from build123d import *

# Parameters (mm, degrees)
F1_DEPTH  = 8.89
F3_DEPTH  = 2.54
F5_DEPTH  = 2.54
F6_W      = 4.75
F6_H      = 6.159577
F8_W      = 4.75
F8_H      = 6.147177
F7_W      = 4.75
F7_H      = 6.147177
F9_W      = 4.75
F9_H      = 6.147177
F10_DEPTH = 6
F11_R     = 1.5
F12_R     = 1.5
F13_R     = 1.5
F14_R     = 1.5
F15_DEPTH = 6
F16_R     = 0.5
F17_DEPTH = 3.5


with BuildPart() as f1:
    # F0 (on Right) → F1 (new body, symmetric)
    with BuildSketch(Plane.YZ):
        Polygon((10.382133, 24.079738), (1.882133, 24.079738), (1, 19.076915), (0, 19.076915), (0, 12.679738), (-8.5, 12.679738), (-9.382133, 7.676915), (-10.382133, 7.676915), (-10.382133, 1.279738), (-18.882133, 1.279738), (-19.764265, -3.723085), (-20.764265, -3.723085), (-20.764265, -10.120262), (-29.264265, -10.120262), (-30.146398, -15.123085), (-31.146398, -15.123085), (-31.146398, -23.920262), (11.753602, -23.920262), (11.753602, 14.92088), align=None)
    extrude(amount=F1_DEPTH, both=True)

    # F2 (on face) → F3 (cut)
    with BuildSketch(Plane(origin=(-8.89, 0, 0), x_dir=(0, -1, 0), z_dir=(-1, 0, 0))):
        Polygon((-11.753602, -23.920262), (0, -23.920262), (0, 12.679738), (0, 19.076915), (-1, 19.076915), (-1.882133, 24.079738), (-10.382133, 24.079738), (-11.753602, 14.92088), align=None)
        Polygon((20.764265, -23.920262), (20.764265, -10.120262), (20.764265, -3.723085), (19.764265, -3.723085), (18.882133, 1.279738), (10.382133, 1.279738), (10.382133, -23.920262), align=None)
    extrude(amount=-F3_DEPTH, mode=Mode.SUBTRACT)

    # F4 (on face) → F5 (cut)
    with BuildSketch(Plane.YZ.offset(8.89)):
        Polygon((-20.764265, -23.920262), (-20.764265, -10.120262), (-29.264265, -10.120262), (-30.146398, -15.123085), (-31.146398, -15.123085), (-31.146398, -23.920262), align=None)
        Polygon((-10.382133, 1.279738), (-10.382133, -23.920262), (0, -23.920262), (0, 12.679738), (-8.5, 12.679738), (-9.382133, 7.676915), (-10.382133, 7.676915), align=None)
    extrude(amount=-F5_DEPTH, mode=Mode.SUBTRACT)

    # F6 (on face) + F8 (on face) + F7 (on face) + F9 (on face) → F10 (cut)
    with BuildSketch(Plane.XZ.offset(31.146398)):
        with Locations((-6.265, -18.452873)):
            Rectangle(F6_W, F6_H)
        with Locations((-1.265, -18.452873)):
            Rectangle(F6_W, F6_H)
        with Locations((3.735, -18.452873)):
            Rectangle(F6_W, F6_H)
    with BuildSketch(Plane.XZ.offset(10.382133)):
        Polygon((-8.64, 7.426915), (-8.64, 1.279738), (-6.35, 1.279738), (-3.89, 1.279738), (-3.89, 7.426915), align=None)
        with Locations((-1.265, 4.353326)):
            Rectangle(F8_W, F8_H)
        with Locations((3.735, 4.353326)):
            Rectangle(F8_W, F8_H)
    with BuildSketch(Plane.XZ.offset(20.764265)):
        with Locations((-3.725, -7.046673)):
            Rectangle(F7_W, F7_H)
        with Locations((1.275, -7.046673)):
            Rectangle(F7_W, F7_H)
        Polygon((3.9, -3.973085), (3.9, -10.120262), (6.35, -10.120262), (8.65, -10.120262), (8.65, -3.973085), align=None)
    with BuildSketch(Plane.XZ):
        with Locations((-3.725, 15.753327)):
            Rectangle(F9_W, F9_H)
        with Locations((1.275, 15.753327)):
            Rectangle(F9_W, F9_H)
        Polygon((3.9, 18.826915), (3.9, 12.679738), (6.35, 12.679738), (8.65, 12.679738), (8.65, 18.826915), align=None)
    extrude(amount=-F10_DEPTH, mode=Mode.SUBTRACT)

    # F11 (on face) + F12 (on face) + F13 (on face) + F14 (on face) → F15 (cut)
    with BuildSketch(Plane.XY.offset(-10.120262)):
        with Locations((-6.265, -27.264265)):
            Circle(F11_R)
        with Locations((-1.265, -27.264265)):
            Circle(F11_R)
        with Locations((3.735, -27.264265)):
            Circle(F11_R)
    with BuildSketch(Plane.XY.offset(1.279738)):
        with Locations((-3.725, -16.882133)):
            Circle(F12_R)
        with Locations((1.275, -16.882133)):
            Circle(F12_R)
        with Locations((6.275, -16.882133)):
            Circle(F12_R)
    with BuildSketch(Plane.XY.offset(12.679738)):
        with Locations((-6.265, -6.5)):
            Circle(F13_R)
        with Locations((-1.265, -6.5)):
            Circle(F13_R)
        with Locations((3.735, -6.5)):
            Circle(F13_R)
    with BuildSketch(Plane.XY.offset(24.079738)):
        with Locations((-3.725, 3.882133)):
            Circle(F14_R)
        with Locations((1.275, 3.882133)):
            Circle(F14_R)
        with Locations((6.275, 3.882133)):
            Circle(F14_R)
    extrude(amount=-F15_DEPTH, mode=Mode.SUBTRACT)

    # F16 (on face) → F17 (join)
    with BuildSketch(Plane(origin=(0, 0, -23.920262), x_dir=(1, 0, 0), z_dir=(0, 0, -1))):
        with Locations((3.81, 26.496398)):
            Circle(F16_R)
        with Locations((-1.27, 26.496398)):
            Circle(F16_R)
        with Locations((-6.35, 26.496398)):
            Circle(F16_R)
        with Locations((6.35, 11.256398)):
            Circle(F16_R)
        with Locations((1.27, 11.256398)):
            Circle(F16_R)
        with Locations((-3.81, 11.256398)):
            Circle(F16_R)
        with Locations((-6.35, 1.096398)):
            Circle(F16_R)
        with Locations((-1.27, 1.096398)):
            Circle(F16_R)
        with Locations((3.81, 1.096398)):
            Circle(F16_R)
        with Locations((6.35, -9.063602)):
            Circle(F16_R)
        with Locations((1.27, -9.063602)):
            Circle(F16_R)
        with Locations((-3.81, -9.063602)):
            Circle(F16_R)
    extrude(amount=F17_DEPTH)


solid = f1.part
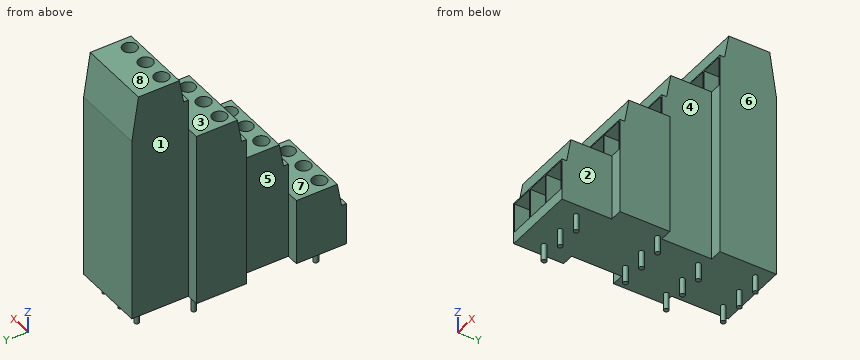
Check sheet for the modelled part. Datum: model origin and axes. Units: mm. Face numbers are marked on the shaded views. A direction names the side the tool comes from. Round coordinates to 2 decimals unless told otherwise and drop trailing zeros. Loops run counter-clockwise (first coordinate to the right, second up) from the corner with the lowest first, then second, coordinate; pieces in that order, holes last. Notation, with made-up numbers: (76, -29) - (82, -29) arc R24 ccw to (82, 3) - close; hole circle Ø5 at (70.25, 7). An arc over 180 degrees is marked (long way). Answer as CSV lines item,"result". Start each with the question number.
Item 1: Section check C-C (z = -20.5). Record the boundary of the cut face in (x, y), and give its area (3 significant figures).
Item 2: Set-up check for the marked faces 1, 2, 3, 4 and 5: record each of +Z, -Z, +X, -X, +Y, -Y from which the full face is reachable in a straight line by a thin tool's end or side.
Item 3: Scan lines: line 1 (X direction, y = -27, z = -16); line 2 (X direction, y = 4.5, z = 16.5); line 3 (Z direction, x = 5.5, y = 2). Record each from-to range of solid material in increasing order. Write a range as [from, to].
Item 4: Section check D-D (z = 6.5). Record the boundary of the cut face in (x, y), and give its area (3 significant figures).
Item 5: Section check A-A (y = -6.5). Record the boundary of the cut face in (x, z) (3 decimals), and give its area (3 significant figures).
Item 6: Depth check by flat-ended pin: P1, Ø1.8, axis at x = -6.26, y = -27.26, coming from the +Z side; P2, Ø4, axis at x = 2.5, y = -29.5, coming from the +Z side; P3, Ø0.5, axis at x = -1, y = 0.5, coming from the +Z side. Enter the tip coordinate at first touch or a pass-through.
Item 7: Section check B-B (z = -5.5). Record the boundary of the cut face in (x, y), and give its area (3 significant figures).
Item 8: Release check for a two-part mould opening along X. For the marked faces 6, 7 and 8 record: +X half, -X half, draft (parallel to the pull), parting line (faces both ways), or undercut.
Report:
1,outline,"(-8.89, -31.15) - (-8.64, -31.15) - (-8.64, -25.15) - (-3.89, -25.15) - (-3.89, -31.15) - (-3.64, -31.15) - (-3.64, -25.15) - (1.11, -25.15) - (1.11, -31.15) - (1.36, -31.15) - (1.36, -25.15) - (6.11, -25.15) - (6.11, -31.15) - (6.35, -31.15) - (6.35, -20.76) - (8.89, -20.76) - (8.89, -10.38) - (6.35, -10.38) - (6.35, 0) - (8.89, 0) - (8.89, 11.75) - (-6.35, 11.75) - (-6.35, 0) - (-8.89, 0) - (-8.89, -10.38) - (-6.35, -10.38) - (-6.35, -20.76) - (-8.89, -20.76) - close"
1,area,"568 mm2"
2,face 1,"+Z, -Z, -X, +Y"
2,face 2,"+Z, -Z, +X, -Y"
2,face 3,"-Y"
2,face 4,"+Z, -Z, +X"
2,face 5,"+Z, -Z, -X"
3,line 1,"x = [-8.89, -8.64], [-3.89, -3.64], [1.11, 1.36], [6.11, 6.35]"
3,line 2,"x = [-6.35, -6.1], [-1.35, -1.1], [3.65, 3.9], [8.65, 8.89]"
3,line 3,"z = [-23.92, 12.68], [18.83, 24.08]"
4,outline,"(-8.89, -10.38) - (-8.64, -10.38) - (-8.64, -4.38) - (-3.89, -4.38) - (-3.89, -10.38) - (-3.64, -10.38) - (-3.64, -4.38) - (1.11, -4.38) - (1.11, -10.38) - (1.36, -10.38) - (1.36, -4.38) - (6.11, -4.38) - (6.11, -10.38) - (6.35, -10.38) - (6.35, 0) - (8.89, 0) - (8.89, 11.75) - (-6.35, 11.75) - (-6.35, 0) - (-8.89, 0) - close"
4,area,"252 mm2"
5,outline,"(-8.89, -23.92) - (6.35, -23.92) - (6.35, 12.68) - (5.235, 12.68) - (5.235, 7.427) - (6.11, 7.427) - (6.11, 1.28) - (1.36, 1.28) - (1.36, 7.427) - (2.235, 7.427) - (2.235, 12.68) - (0.235, 12.68) - (0.235, 7.427) - (1.11, 7.427) - (1.11, 1.28) - (-3.64, 1.28) - (-3.64, 7.427) - (-2.765, 7.427) - (-2.765, 12.68) - (-4.765, 12.68) - (-4.765, 7.427) - (-3.89, 7.427) - (-3.89, 1.28) - (-8.64, 1.28) - (-8.64, 7.427) - (-7.765, 7.427) - (-7.765, 12.68) - (-8.89, 12.68) - close"
5,area,"423 mm2"
6,P1,"stops at z = -21.53"
6,P2,"stops at z = -10.12"
6,P3,"stops at z = 19.08"
7,outline,"(-8.89, -10.38) - (-6.35, -10.38) - (-6.35, -20.76) - (-6.1, -20.76) - (-6.1, -14.76) - (-1.35, -14.76) - (-1.35, -20.76) - (-1.1, -20.76) - (-1.1, -14.76) - (3.65, -14.76) - (3.65, -20.76) - (3.9, -20.76) - (3.9, -14.76) - (8.65, -14.76) - (8.65, -20.76) - (8.89, -20.76) - (8.89, -10.38) - (6.35, -10.38) - (6.35, 0) - (8.89, 0) - (8.89, 11.75) - (-6.35, 11.75) - (-6.35, 0) - (-8.89, 0) - close"
7,area,"410 mm2"
8,face 6,"+X half"
8,face 7,"undercut"
8,face 8,"draft"
